from build123d import *

# Parameters (mm, degrees)
SKETCH_1_R               = 9.97
EXTRUDE_1_DEPTH          = 25
FILLET_1_R               = 0.5
SKETCH_2_W               = 1.8
SKETCH_2_H               = 2.1
FILLET_2_R               = 0.2
CUT_EXTRUDE_1_DEPTH      = 29.701947669
CUT_EXTRUDE_1_DEPTH_BACK = 29.701947669
SKETCH_4_R               = 2
CHAMFER_1_SIZE           = 0.5
CUT_EXTRUDE_4_DEPTH      = 29.701947748
CUT_EXTRUDE_4_DEPTH_BACK = 29.701947748
SKETCH_7_W               = 12
SKETCH_7_H               = 5
CUT_EXTRUDE_START        = 5
SKETCH_8_R               = 7.5
CUT_EXTRUDE_5_DEPTH      = 24


with BuildPart() as part:
    # Sketch 1 → Extrude 1 (new body)
    with BuildSketch(Plane(origin=(0, 0, 0), x_dir=(1, 0, 0), z_dir=(0, 1, 0))):
        with Locations(Location((0, 0, 0), (0, 0, 270))):
            Circle(SKETCH_1_R)
    extrude(amount=EXTRUDE_1_DEPTH)

    # Fillet 1
    fillet_1_edges = [part.edges().sort_by_distance(p)[0] for p in [
        (0, 25, -9.97),
    ]]
    fillet(fillet_1_edges, radius=FILLET_1_R)

    # Sketch 2 → Cut-Revolve 1 (revolve, cut)
    with BuildSketch(Plane.XY, mode=Mode.PRIVATE) as cut_revolve_1_sk:
        with Locations((-9.07, 21.95)):
            Rectangle(SKETCH_2_W, SKETCH_2_H)
        with Locations((-9.07, 17.35)):
            Rectangle(SKETCH_2_W, SKETCH_2_H)
    revolve(cut_revolve_1_sk.sketch.rotate(Axis((0, 0, 0), (0, 1, 0)), 270), axis=Axis((0, 0, 0), (0, 1, 0)), mode=Mode.SUBTRACT)

    # Fillet 2
    fillet_2_edges = [part.edges().sort_by_distance(p)[0] for p in [
        (0, 20.9, 8.17),
        (0, 23, 8.17),
        (0, 16.3, 8.17),
        (0, 18.4, 8.17),
    ]]
    fillet(fillet_2_edges, radius=FILLET_2_R)

    # Sketch 4 → Cut-Extrude 1 (cut, two sides: drawn at the far end of the back side and taken through both)
    with BuildSketch(Plane.XY.offset(-CUT_EXTRUDE_1_DEPTH_BACK)):
        with Locations((0, 8.5)):
            Circle(SKETCH_4_R)
    extrude(amount=CUT_EXTRUDE_1_DEPTH + CUT_EXTRUDE_1_DEPTH_BACK, mode=Mode.SUBTRACT)

    # Chamfer 1
    chamfer_1_edges = [part.edges().sort_by_distance(p)[0] for p in [
        (0, 0, -9.97),
    ]]
    chamfer(chamfer_1_edges, length=CHAMFER_1_SIZE)

    # Sketch 7 → Cut-Extrude 4 (cut, two sides: drawn at the far end of the back side and taken through both)
    with BuildSketch(Plane(origin=(0, 0, 0), x_dir=(0, 0, -1), z_dir=(1, 0, 0)).offset(-CUT_EXTRUDE_4_DEPTH_BACK)):
        with Locations((0, 2.5)):
            Rectangle(SKETCH_7_W, SKETCH_7_H)
    extrude(amount=CUT_EXTRUDE_4_DEPTH + CUT_EXTRUDE_4_DEPTH_BACK, mode=Mode.SUBTRACT)

    # Sketch 8 → Cut-Extrude 5 (cut)
    with BuildSketch(Plane.XZ.offset(-5).offset(CUT_EXTRUDE_START)):
        with Locations(Location((0, 0, 0), (0, 0, 270))):
            Circle(SKETCH_8_R)
    extrude(amount=-CUT_EXTRUDE_5_DEPTH, mode=Mode.SUBTRACT)


solid = part.part
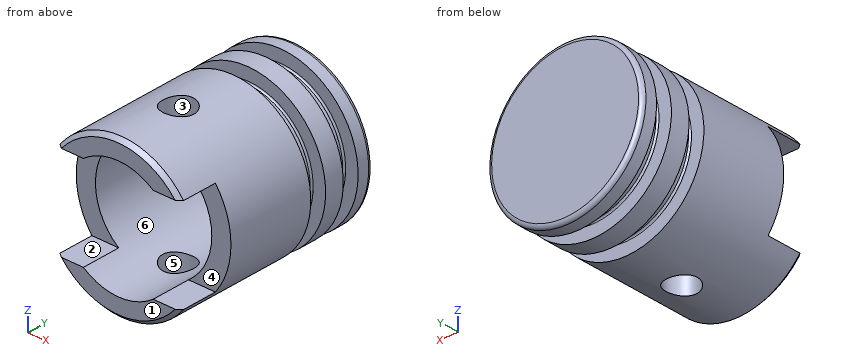
Read the model definition and answer for the solid it produces. Units are mm, in the model's axes. Face numbers are marked on the shaded views. A direction names the side the tool comes from. Give positions to 0.01 mm unless a question says otherwise; leave off trailing zeros. Write each loop counter-clockwise with the first axis right and the second up, starting at its lowest first coordinate (ties: lowest second). Pieces come first, ordered by that corner, then holes. Notation, with made-up numbers: (5.5, 80.5) - (63.5, 80.5) arc R22 ccw to (63.5, 115.5) - close; hole circle Ø1 at (88, 56.25). An arc over 180 degrees is marked (long way). Answer in a Markdown table with one row per item. Add a question column.
Item 1: Section A-A, the plane y = 2 is taken. Write down the section's boundary in (x, z), and give its area (3 significant figures).
Item 2: Section C-C, the plane x = 0 is taken. Count the separate pieces of the cut face and the enclosed holes in it, and give its area (3 significant figures).
Item 3: Section D-D, the plane y = 8.5 is taken. Write down the section's boundary in (x, z), and give its area (3 significant figures).
Item 4: Flat-ended cylindrical pins translate along their axes: P1, Ø4, axis at y = 7, z = -3.5, coming from the +X side; P2, Ø10, axis at x = -5.5, y = 3.5, coming from the +Z side; P3, Ø1.7, axis at x = 7, y = 2.5, coming from the -Z side; P4, Ø3.5, axis at x = 0, y = 8.5, coming from the -Z side. Find the tip coordinate at first contact, or state that the pin passes through.
Item 5: Find the intervals of material crossed by L1, parallel to Y at x = 0, z = 9.15; L2, parallel to Y at x = 6.5, z = -5.25; L3, parallel to Y at x = 4.25, z = 7.5, in increasing order.
Item 6: A tool of negligible diameter and unlimited length cuts with its end or side. For the marked faces 4, 5 and 6, from which of +Z, -Z, +X, -X, +Y, -Y can it reach the whole face along a straight path? Write none if from no direction.
Item 7: Determine the mould class of the marked faces 1, 2 and 3 for opening direction Y: pulls with the +Y half, pulls with the -Y half, needs draft (parallel to the pull), parting line crosses it, or undercut.
Recorded:
| question | item | result |
|---|---|---|
| 1 | outline | (-7.96, -6) arc R9.97 ccw to (7.96, -6) - (4.5, -6) arc R7.5 cw to (-4.5, -6) - close; (-7.96, 6) - (-4.5, 6) arc R7.5 cw to (4.5, 6) - (7.96, 6) arc R9.97 ccw to start |
| 1 | area | 70.0 mm2 |
| 2 | separate pieces | 3 |
| 2 | enclosed holes | 0 |
| 2 | area | 103 mm2 |
| 3 | outline | (-2, -9.77) - (-2, -7.23) arc R7.5 cw to (-2, 7.23) - (-2, 9.77) arc R9.97 ccw to start; (2, -9.77) arc R9.97 ccw to (2, 9.77) - (2, 7.23) arc R7.5 cw to (2, -7.23) - close |
| 3 | area | 116 mm2 |
| 4 | P1 | stops at x = 9.86 |
| 4 | P2 | stops at z = 9.96 |
| 4 | P3 | stops at z = -7.85 |
| 4 | P4 | passes through |
| 5 | L1 | y = 0 to 6.5, 10.5 to 16.3, 18.4 to 20.9, 23 to 25 |
| 5 | L2 | y = 5 to 16.3, 18.4 to 20.9, 23 to 25 |
| 5 | L3 | y = 0 to 16.3, 18.4 to 20.9, 23 to 25 |
| 6 | face 4 | +X, -X, -Y |
| 6 | face 5 | +Z, -Z |
| 6 | face 6 | -Y |
| 7 | face 1 | pulls with the -Y half |
| 7 | face 2 | needs draft |
| 7 | face 3 | undercut |
